Design review of the part built by this model. Coordinates are the model's own, in mm. A direction names the side the tool comes from. Round coordinates to 2 decimals unless told otherwise and drop trailing zeros. Write item = value, one per line. Start each with the question number.
Item 1: To check wall thickness, follow L1, parallel to X at y = -1, z = 2; L2, parallel to X at y = -13, z = 8.5; L3, parallel to X at y = 5.5, z = 13. State the ranges of each line that lie inside material, in increasing order.
Item 2: For pin 1 Ø10 at (y, z) = (6, 55.5) entering from -X; pin 2 Ø4 at (y, z) = (-3.5, 50.5) entering from -X; pin 3 Ø0.5 at (x, z) = (12.5, 11) entering from -Y, all flat-tipped, find the tip position at first contact; note any pin that passes through.
Item 3: Add section A-A, the plane z = 5.5. State how many separate pieces and enclosed holes the cut face has, then the cut area to 3 significant figures.
Item 4: Machinability: for faces 1 (the flat face through (0, -5, 25.4)), 2 (the cylindrical face through (7.874, -2.48, 5.151)), which of the approach directions +Z, -Z, +X, -X, +Y, -Y give a long, thin tool a straight path to every point of the face, cutting with its end or side? Answer none if there is none.
Item 5: Mouldability with a two-part tool opening along Y and no side actions: class faces 3 (the flat face through (4.4, -10.1, 25.4)), 4 (the flat face through (-12.05, 8.04, 12.88)) as released by +Y, released by -Y, zero draft, split by the parting line, or undercut.
from build123d import *

# Parameters (mm, degrees)
SKETCH1_R           = 15.24
BOSS_EXTRUDE1_DEPTH = 25.4
CUT_EXTRUDE1_DEPTH  = 25.4
SKETCH3_R           = 6.35
BOSS_EXTRUDE2_DEPTH = 25.4
CUT_EXTRUDE2_DEPTH  = 25.4
SKETCH6_R           = 10.795
SKETCH6_R_2         = 8.255
CUT_EXTRUDE3_DEPTH  = 10.16
CUT_EXTRUDE4_START  = -10.16
SKETCH7_R           = 10.795
SKETCH7_R_2         = 8.255
CUT_EXTRUDE4_DEPTH  = 10.16
SKETCH8_R           = 2.54
BOSS_EXTRUDE3_DEPTH = 12.7
BOSS_EXTRUDE4_START = 3.81
SKETCH9_R           = 2.54
BOSS_EXTRUDE4_DEPTH = 3.81


with BuildPart() as part:
    # Sketch1 → Boss-Extrude1 (new body)
    with BuildSketch(Plane.XY):
        Circle(SKETCH1_R)
    extrude(amount=BOSS_EXTRUDE1_DEPTH)

    # Sketch2 → Cut-Extrude1 (cut)
    with BuildSketch(Plane.XY.offset(25.4)):
        Polygon((2.595770068, 13.468134012), (4.324370212, 15.463044922), (1.732426613, 15.962601105), align=None)
        Polygon((0, 13.716), (1.319822715, 16.002), (-1.319822715, 16.002), align=None)
        Polygon((5.097722242, 12.733494569), (7.172623702, 14.365215113), (4.722061529, 15.346272216), align=None)
        Polygon((7.415429452, 11.538633456), (9.761639883, 12.748189001), (7.541028839, 14.175289064), align=None)
        Polygon((9.465123721, 9.926736067), (11.997844965, 10.670410123), (10.087443718, 12.491974033), align=None)
        Polygon((11.172723758, 7.956060572), (13.80041667, 8.206974822), (12.269272099, 10.357166512), align=None)
        Polygon((12.476512448, 5.697832318), (15.10420536, 5.446918068), (14.007657019, 7.848024008), align=None)
        Polygon((13.329367471, 3.233669559), (15.862088715, 2.489995503), (15.239768718, 5.055233469), align=None)
        Polygon((13.700464424, 0.652633557), (16.046674855, -0.556921987), (15.921075468, 2.079733621), align=None)
        Polygon((13.576390897, -1.951990322), (15.651292357, -3.583710865), (16.026953069, -0.970933219), align=None)
        Polygon((12.961631229, -4.486064185), (14.690231374, -6.480975096), (15.553574829, -3.986508002), align=None)
        Polygon((11.878404438, -6.858), (13.198227154, -9.144), (14.518049869, -6.858), align=None)
        Polygon((10.365861162, -8.982069827), (11.229204617, -11.47653692), (12.957804761, -9.481626009), align=None)
        Polygon((8.478668655, -10.781504247), (8.854329368, -13.394281894), (10.929230827, -11.76256135), align=None)
        Polygon((6.285034972, -12.191267014), (6.159435585, -14.827922622), (8.505646016, -13.618367077), align=None)
        Polygon((3.86424375, -13.160405626), (3.241923753, -15.725643592), (5.774644996, -14.981969536), align=None)
        Polygon((1.30378869, -13.65389289), (0.207240349, -16.05499883), (2.834933261, -15.80408458), align=None)
        Polygon((-1.30378869, -13.65389289), (-2.834933261, -15.80408458), (-0.207240349, -16.05499883), align=None)
        Polygon((-3.86424375, -13.160405626), (-5.774644996, -14.981969536), (-3.241923753, -15.725643592), align=None)
        Polygon((-6.285034972, -12.191267014), (-8.505646016, -13.618367077), (-6.159435585, -14.827922622), align=None)
        Polygon((-8.478668655, -10.781504247), (-10.929230827, -11.76256135), (-8.854329368, -13.394281894), align=None)
        Polygon((-10.365861162, -8.982069827), (-12.957804761, -9.481626009), (-11.229204617, -11.47653692), align=None)
        Polygon((-11.878404438, -6.858), (-14.518049869, -6.858), (-13.198227154, -9.144), align=None)
        Polygon((-12.961631229, -4.486064185), (-15.553574829, -3.986508002), (-14.690231374, -6.480975096), align=None)
        Polygon((-13.576390897, -1.951990322), (-16.026953069, -0.970933219), (-15.651292357, -3.583710865), align=None)
        Polygon((-13.700464424, 0.652633557), (-15.921075468, 2.079733621), (-16.046674855, -0.556921987), align=None)
        Polygon((-13.329367471, 3.233669559), (-15.239768718, 5.055233469), (-15.862088715, 2.489995503), align=None)
        Polygon((-12.476512448, 5.697832318), (-14.007657019, 7.848024008), (-15.10420536, 5.446918068), align=None)
        Polygon((-11.172723758, 7.956060572), (-12.269272099, 10.357166512), (-13.80041667, 8.206974822), align=None)
        Polygon((-9.465123721, 9.926736067), (-10.087443718, 12.491974033), (-11.997844965, 10.670410123), align=None)
        Polygon((-7.415429452, 11.538633456), (-7.541028839, 14.175289064), (-9.761639883, 12.748189001), align=None)
        Polygon((-5.097722242, 12.733494569), (-4.722061529, 15.346272216), (-7.172623702, 14.365215113), align=None)
        Polygon((-2.595770068, 13.468134012), (-1.732426613, 15.962601105), (-4.324370212, 15.463044922), align=None)
    extrude(amount=-CUT_EXTRUDE1_DEPTH, mode=Mode.SUBTRACT)

    # Sketch3 → Boss-Extrude2 (add)
    with BuildSketch(Plane.XY.offset(25.4)):
        Circle(SKETCH3_R)
    extrude(amount=BOSS_EXTRUDE2_DEPTH)

    # Sketch5 → Cut-Extrude2 (cut)
    with BuildSketch(Plane.XY.offset(50.8)):
        Polygon((1.983716455, 4.119229664), (4.528190095, 5.854022418), (1.75357868, 7.190204852), align=None)
        Polygon((0, 4.572), (1.539793168, 7.239), (-1.539793168, 7.239), align=None)
        Polygon((3.574533538, 2.850595374), (6.619723439, 3.3095839), (4.699632764, 5.717301451), align=None)
        Polygon((4.457370414, 1.01736571), (7.40013937, 0.109641703), (6.714866942, 3.112016379), align=None)
        Polygon((4.457370414, -1.01736571), (6.714866942, -3.112016379), (7.40013937, -0.109641703), align=None)
        Polygon((3.574533538, -2.850595374), (4.699632764, -5.717301451), (6.619723439, -3.3095839), align=None)
        Polygon((1.983716455, -4.119229664), (1.75357868, -7.190204852), (4.528190095, -5.854022418), align=None)
        Polygon((0, -4.572), (-1.539793168, -7.239), (1.539793168, -7.239), align=None)
        Polygon((-1.983716455, -4.119229664), (-4.528190095, -5.854022418), (-1.75357868, -7.190204852), align=None)
        Polygon((-3.574533538, -2.850595374), (-6.619723439, -3.3095839), (-4.699632764, -5.717301451), align=None)
        Polygon((-4.457370414, -1.01736571), (-7.40013937, -0.109641703), (-6.714866942, -3.112016379), align=None)
        Polygon((-4.457370414, 1.01736571), (-6.714866942, 3.112016379), (-7.40013937, 0.109641703), align=None)
        Polygon((-3.574533538, 2.850595374), (-4.699632764, 5.717301451), (-6.619723439, 3.3095839), align=None)
        Polygon((-1.983716455, 4.119229664), (-1.75357868, 7.190204852), (-4.528190095, 5.854022418), align=None)
    extrude(amount=-CUT_EXTRUDE2_DEPTH, mode=Mode.SUBTRACT)

    # Sketch6 → Cut-Extrude3 (cut)
    with BuildSketch(Plane.XY.offset(25.4)):
        Circle(SKETCH6_R)
        Circle(SKETCH6_R_2, mode=Mode.SUBTRACT)
    extrude(amount=-CUT_EXTRUDE3_DEPTH, mode=Mode.SUBTRACT)

    # Sketch7 → Cut-Extrude4 (cut)
    with BuildSketch(Plane(origin=(0, 0, 0), x_dir=(-1, 0, 0), z_dir=(0, 0, -1)).offset(CUT_EXTRUDE4_START)):
        with Locations(Location((0, 0, 0), (0, 0, 180))):
            Circle(SKETCH7_R)
        with Locations(Location((0, 0, 0), (0, 0, 180))):
            Circle(SKETCH7_R_2, mode=Mode.SUBTRACT)
    extrude(amount=CUT_EXTRUDE4_DEPTH, mode=Mode.SUBTRACT)

    # Sketch8 → Boss-Extrude3 (add)
    with BuildSketch(Plane.XY.offset(50.8)):
        Circle(SKETCH8_R)
    extrude(amount=BOSS_EXTRUDE3_DEPTH)

    # Sketch9 → Boss-Extrude4 (add)
    with BuildSketch(Plane(origin=(0, 0, 0), x_dir=(-1, 0, 0), z_dir=(0, 0, -1)).offset(BOSS_EXTRUDE4_START)):
        with Locations(Location((0, 0, 0), (0, 0, 180))):
            Circle(SKETCH9_R)
    extrude(amount=-BOSS_EXTRUDE4_DEPTH)


solid = part.part
Result set:
q1.L1 = -15.21 to -10.75, -8.19 to 8.19, 10.75 to 15.21
q1.L2 = -7.95 to -7.54, -6.25 to 6.25, 7.54 to 7.95
q1.L3 = -14.21 to 14.21
q2.pin_1 = -4.29
q2.pin_2 = -5.9
q2.pin_3 = -9.07
q3.separate_pieces = 2
q3.enclosed_holes = 1
q3.area = 534 mm²
q4.face_1 = +Z
q4.face_2 = -Z
q5.face_3 = zero draft
q5.face_4 = undercut
